Geometry: final body of the model. Coordinates: model frame, mm. Give positions to 0.01 mm unless a question says otherwise; leave off trailing zeros. Write each loop counter-clockwise with the first axis right and the second up, starting at its lowest first coordinate (ties: lowest second). Pieces come first, ordered by that corner, then holes. Notation, with made-up numbers: (-13, -10.5) -> (32, -10.5) arc R28 cw to (32, 27.5) -> close; hole circle Ø2 at (35, -36.75). An arc over 180 degrees is marked (long way). Answer as a JSON object with one key per item and string values. Group by question number.
(1) Section query B-B on y = 0.85. State how many separate pieces and enclosed holes the cut face has, plus the area to 3 significant figures.
(2) Section query A-A on z = 105. Output: boundary loops of the cut face in (x, y) (3 decimals), plus the area to 3 significant figures.
(3) Material intervals for probe 1 along Z at (x, y) = (-112, 0.9); probe 2 along Z at (x, y) = (-72, 1); probe 3 along X at (y, z) = (0.7, -174), sorted ascending.
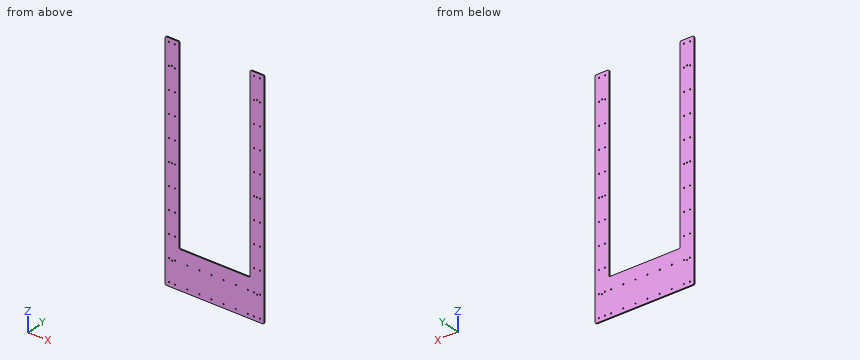
from build123d import *

# Parameters (mm, degrees)
SKETCH1_R           = 1.6
BOSS_EXTRUDE1_DEPTH = 3.175
FILLET1_R           = 3


with BuildPart() as part:
    # Sketch1 → Boss-Extrude1 (new body)
    with BuildSketch(Plane(origin=(0, 0, 0), x_dir=(1, 0, 0), z_dir=(0, 1, 0))):
        Polygon((-130, -300), (-94, -300), (-94, 200), (94, 200), (94, -300), (130, -300), (130, 300), (-130, 300), align=None)
        with Locations(Location((120, 290, 0), (0, 0, 270))):
            Circle(SKETCH1_R, mode=Mode.SUBTRACT)
        with Locations(Location((120, 232, 0), (0, 0, 270))):
            Circle(SKETCH1_R, mode=Mode.SUBTRACT)
        with Locations(Location((120, 174, 0), (0, 0, 270))):
            Circle(SKETCH1_R, mode=Mode.SUBTRACT)
        with Locations(Location((120, 116, 0), (0, 0, 270))):
            Circle(SKETCH1_R, mode=Mode.SUBTRACT)
        with Locations(Location((120, 58, 0), (0, 0, 270))):
            Circle(SKETCH1_R, mode=Mode.SUBTRACT)
        with Locations(Location((120, 0, 0), (0, 0, 270))):
            Circle(SKETCH1_R, mode=Mode.SUBTRACT)
        with Locations(Location((120, -58, 0), (0, 0, 270))):
            Circle(SKETCH1_R, mode=Mode.SUBTRACT)
        with Locations(Location((120, -116, 0), (0, 0, 270))):
            Circle(SKETCH1_R, mode=Mode.SUBTRACT)
        with Locations(Location((120, -174, 0), (0, 0, 270))):
            Circle(SKETCH1_R, mode=Mode.SUBTRACT)
        with Locations(Location((120, -232, 0), (0, 0, 270))):
            Circle(SKETCH1_R, mode=Mode.SUBTRACT)
        with Locations(Location((120, -290, 0), (0, 0, 270))):
            Circle(SKETCH1_R, mode=Mode.SUBTRACT)
        with Locations(Location((-120, 232, 0), (0, 0, 90))):
            Circle(SKETCH1_R, mode=Mode.SUBTRACT)
        with Locations(Location((-120, -290, 0), (0, 0, 90))):
            Circle(SKETCH1_R, mode=Mode.SUBTRACT)
        with Locations(Location((-120, -232, 0), (0, 0, 90))):
            Circle(SKETCH1_R, mode=Mode.SUBTRACT)
        with Locations(Location((-120, -174, 0), (0, 0, 90))):
            Circle(SKETCH1_R, mode=Mode.SUBTRACT)
        with Locations(Location((-120, -116, 0), (0, 0, 90))):
            Circle(SKETCH1_R, mode=Mode.SUBTRACT)
        with Locations(Location((-120, -58, 0), (0, 0, 90))):
            Circle(SKETCH1_R, mode=Mode.SUBTRACT)
        with Locations(Location((-120, 0, 0), (0, 0, 90))):
            Circle(SKETCH1_R, mode=Mode.SUBTRACT)
        with Locations(Location((-120, 58, 0), (0, 0, 90))):
            Circle(SKETCH1_R, mode=Mode.SUBTRACT)
        with Locations(Location((-120, 116, 0), (0, 0, 90))):
            Circle(SKETCH1_R, mode=Mode.SUBTRACT)
        with Locations(Location((-120, 174, 0), (0, 0, 90))):
            Circle(SKETCH1_R, mode=Mode.SUBTRACT)
        with Locations(Location((-120, 290, 0), (0, 0, 90))):
            Circle(SKETCH1_R, mode=Mode.SUBTRACT)
        with Locations(Location((112, 235, 0), (0, 0, 270))):
            Circle(SKETCH1_R, mode=Mode.SUBTRACT)
        with Locations(Location((-112, 235, 0), (0, 0, 90))):
            Circle(SKETCH1_R, mode=Mode.SUBTRACT)
        with Locations(Location((112, -235, 0), (0, 0, 90))):
            Circle(SKETCH1_R, mode=Mode.SUBTRACT)
        with Locations(Location((-112, -235, 0), (0, 0, 270))):
            Circle(SKETCH1_R, mode=Mode.SUBTRACT)
        with Locations(Location((104, 290, 0), (0, 0, 270))):
            Circle(SKETCH1_R, mode=Mode.SUBTRACT)
        with Locations(Location((104, 232, 0), (0, 0, 270))):
            Circle(SKETCH1_R, mode=Mode.SUBTRACT)
        with Locations(Location((104, 174, 0), (0, 0, 270))):
            Circle(SKETCH1_R, mode=Mode.SUBTRACT)
        with Locations(Location((104, 116, 0), (0, 0, 270))):
            Circle(SKETCH1_R, mode=Mode.SUBTRACT)
        with Locations(Location((104, 58, 0), (0, 0, 270))):
            Circle(SKETCH1_R, mode=Mode.SUBTRACT)
        with Locations(Location((104, 0, 0), (0, 0, 270))):
            Circle(SKETCH1_R, mode=Mode.SUBTRACT)
        with Locations(Location((104, -58, 0), (0, 0, 270))):
            Circle(SKETCH1_R, mode=Mode.SUBTRACT)
        with Locations(Location((104, -116, 0), (0, 0, 270))):
            Circle(SKETCH1_R, mode=Mode.SUBTRACT)
        with Locations(Location((104, -174, 0), (0, 0, 270))):
            Circle(SKETCH1_R, mode=Mode.SUBTRACT)
        with Locations(Location((104, -232, 0), (0, 0, 270))):
            Circle(SKETCH1_R, mode=Mode.SUBTRACT)
        with Locations(Location((104, -290, 0), (0, 0, 270))):
            Circle(SKETCH1_R, mode=Mode.SUBTRACT)
        with Locations(Location((-104, -290, 0), (0, 0, 90))):
            Circle(SKETCH1_R, mode=Mode.SUBTRACT)
        with Locations(Location((-104, -232, 0), (0, 0, 90))):
            Circle(SKETCH1_R, mode=Mode.SUBTRACT)
        with Locations(Location((-104, -174, 0), (0, 0, 90))):
            Circle(SKETCH1_R, mode=Mode.SUBTRACT)
        with Locations(Location((-104, -116, 0), (0, 0, 90))):
            Circle(SKETCH1_R, mode=Mode.SUBTRACT)
        with Locations(Location((-104, -58, 0), (0, 0, 90))):
            Circle(SKETCH1_R, mode=Mode.SUBTRACT)
        with Locations(Location((-104, 0, 0), (0, 0, 90))):
            Circle(SKETCH1_R, mode=Mode.SUBTRACT)
        with Locations(Location((-104, 58, 0), (0, 0, 90))):
            Circle(SKETCH1_R, mode=Mode.SUBTRACT)
        with Locations(Location((-104, 116, 0), (0, 0, 90))):
            Circle(SKETCH1_R, mode=Mode.SUBTRACT)
        with Locations(Location((-104, 174, 0), (0, 0, 90))):
            Circle(SKETCH1_R, mode=Mode.SUBTRACT)
        with Locations(Location((-104, 232, 0), (0, 0, 90))):
            Circle(SKETCH1_R, mode=Mode.SUBTRACT)
        with Locations(Location((-104, 290, 0), (0, 0, 90))):
            Circle(SKETCH1_R, mode=Mode.SUBTRACT)
        with Locations(Location((112, 0, 0), (0, 0, 270))):
            Circle(SKETCH1_R, mode=Mode.SUBTRACT)
        with Locations(Location((-112, 0, 0), (0, 0, 90))):
            Circle(SKETCH1_R, mode=Mode.SUBTRACT)
        with Locations(Location((-72, 290, 0), (0, 0, 90))):
            Circle(SKETCH1_R, mode=Mode.SUBTRACT)
        with Locations(Location((-40, 290, 0), (0, 0, 90))):
            Circle(SKETCH1_R, mode=Mode.SUBTRACT)
        with Locations(Location((-8, 290, 0), (0, 0, 90))):
            Circle(SKETCH1_R, mode=Mode.SUBTRACT)
        with Locations(Location((24, 290, 0), (0, 0, 90))):
            Circle(SKETCH1_R, mode=Mode.SUBTRACT)
        with Locations(Location((56, 290, 0), (0, 0, 90))):
            Circle(SKETCH1_R, mode=Mode.SUBTRACT)
        with Locations(Location((88, 290, 0), (0, 0, 90))):
            Circle(SKETCH1_R, mode=Mode.SUBTRACT)
        with Locations(Location((-72, 232, 0), (0, 0, 90))):
            Circle(SKETCH1_R, mode=Mode.SUBTRACT)
        with Locations(Location((-40, 232, 0), (0, 0, 90))):
            Circle(SKETCH1_R, mode=Mode.SUBTRACT)
        with Locations(Location((-8, 232, 0), (0, 0, 90))):
            Circle(SKETCH1_R, mode=Mode.SUBTRACT)
        with Locations(Location((24, 232, 0), (0, 0, 90))):
            Circle(SKETCH1_R, mode=Mode.SUBTRACT)
        with Locations(Location((56, 232, 0), (0, 0, 90))):
            Circle(SKETCH1_R, mode=Mode.SUBTRACT)
        with Locations(Location((88, 232, 0), (0, 0, 90))):
            Circle(SKETCH1_R, mode=Mode.SUBTRACT)
    extrude(amount=BOSS_EXTRUDE1_DEPTH)

    # Fillet1
    fillet1_edges = [part.edges().sort_by_distance(p)[0] for p in [
        (130, 1.5875, 300),
        (94, 1.5875, 300),
        (94, 1.5875, -200),
        (-94, 1.5875, -200),
        (-94, 1.5875, 300),
        (-130, 1.5875, 300),
        (-130, 1.5875, -300),
        (130, 1.5875, -300),
    ]]
    fillet(fillet1_edges, radius=FILLET1_R)


solid = part.part
Answer list:
{
 "1": {"separate pieces": "1", "enclosed holes": "62", "area": "61,500 mm2"},
 "2": {"outline": "(-130, 0) -> (-94, 0) -> (-94, 3.175) -> (-130, 3.175) -> close; (94, 0) -> (130, 0) -> (130, 3.175) -> (94, 3.175) -> close", "area": "229 mm2"},
 "3": {"probe 1": "-300 to -236.6, -233.4 to -1.6, 1.6 to 233.4, 236.6 to 300", "probe 2": "-300 to -291.6, -288.4 to -233.6, -230.4 to -200", "probe 3": "-130 to -121.6, -118.4 to -105.6, -102.4 to -94, 94 to 102.4, 105.6 to 118.4, 121.6 to 130"}
}
